Read the model definition and answer for the solid it produces. Units are mm, in the model's axes. Coordinates: 2 decimals unless noted, no trailing zeros. Order: outer loops, then holes, each group sorted by start corner. A loop starts at its lowest first (then second) coordinate and runs counter-clockwise, first axis right, second up. Notation, with made-up numbers: M 43,86 L 52,86 A28 cw 52,124 Z; hole C 40.25,3 d7. An arc over 180 degrees is marked long. One line per question, with ' | ' between items. Start each with the question number.
1) Find section D-D, the plane x = 5.75. Write down the section's boundary in (y, z).
2) Given P1, Ø4, axis at y = 4.5, z = -10, coming from the +X side; P2, Ø3, axis at x = -4.5, z = 9.5, coming from the -Y side; P3, Ø4, axis at y = 4, z = -4.5, coming from the -X side, each flat-ended and moving along its own axis, determine where each tip first touches the part or whether it passes through.
3) Find section B-B, the plane x = 0. Write down the section's boundary in (y, z), plus the area to 3 significant figures.
4) Find section C-C, the plane z = 10. Write down the section's boundary in (x, y), plus the area to 3 significant figures.
5) Consider probe 1 along Y at (x, z) = (0.9, -24); probe 2 along X at (y, z) = (1.5, 19); probe 3 along Z at (x, y) = (-0.25, 5.75). Determine where each line is inside the solid, lowest interval first.
6) Find section A-A, the plane z = -24. Write down the section's boundary in (x, y), plus the area to 3 significant figures.
from build123d import *

# Parameters (mm, degrees)
SKETCH1_W           = 4
SKETCH1_H           = 60
BOSS_EXTRUDE1_DEPTH = 8
SKETCH2_R           = 2.5
CUT_EXTRUDE1_DEPTH  = 8
FILLET1_R           = 3
SKETCH3_R           = 7.5
BOSS_EXTRUDE2_DEPTH = 4
BOSS_EXTRUDE3_DEPTH = 4


with BuildPart() as part:
    # Sketch1 → Boss-Extrude1 (new body)
    with BuildSketch(Plane(origin=(0, 0, 0), x_dir=(1, 0, 0), z_dir=(0, 1, 0))):
        Rectangle(SKETCH1_W, SKETCH1_H)
    extrude(amount=BOSS_EXTRUDE1_DEPTH)

    # Sketch2 → Cut-Extrude1 (cut)
    with BuildSketch(Plane.ZY.offset(2)):
        with Locations((-24, 4)):
            Circle(SKETCH2_R)
    extrude(amount=-CUT_EXTRUDE1_DEPTH, mode=Mode.SUBTRACT)

    # Fillet1
    fillet1_edges = [part.edges().sort_by_distance(p)[0] for p in [
        (0, 0, -30),
        (0, 8, -30),
    ]]
    fillet(fillet1_edges, radius=FILLET1_R)

    # Sketch3 → Boss-Extrude2 (add)
    with BuildSketch(Plane.XZ):
        with Locations((0, 30)):
            Circle(SKETCH3_R)
    extrude(amount=-BOSS_EXTRUDE2_DEPTH)

    # Sketch4 → Boss-Extrude3 (add)
    with BuildSketch(Plane(origin=(2, 0, 0), x_dir=(0, 0, -1), z_dir=(1, 0, 0))):
        Polygon((-30, 4), (-36.351721889, 4), (-30, 8), align=None)
    extrude(amount=-BOSS_EXTRUDE3_DEPTH)


solid = part.part
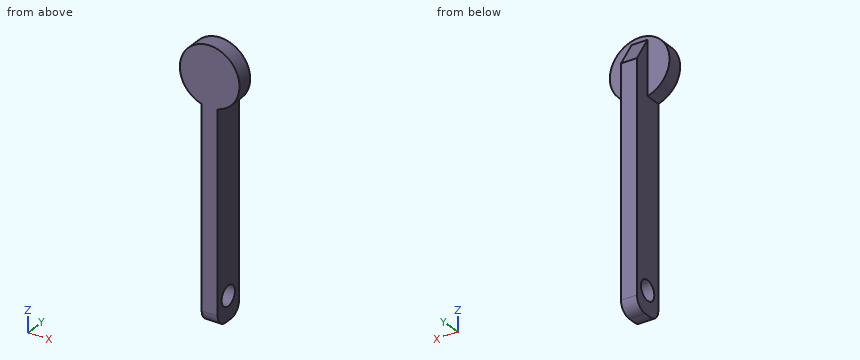
Report:
1) outline: M 0,25.18 L 4,25.18 L 4,34.82 L 0,34.82 Z
2) P1: stops at x = 2 | P2: passes through | P3: stops at x = -2
3) outline: M 0,-27 A3 ccw 3,-30 L 5,-30 A3 ccw 8,-27 L 8,30 L 4,36.35 L 4,37.5 L 0,37.5 Z; hole C 4,-24 d5 | area: 499 mm^2
4) outline: M -2,0 L 2,0 L 2,8 L -2,8 Z | area: 32.0 mm^2
5) probe 1: y = 0 to 1.5, 6.5 to 8 | probe 2: x = -2 to 2 | probe 3: z = -29.9 to -25.79, -22.21 to 33.57
6) outline: M -2,0 L 2,0 L 2,1.5 L -2,1.5 Z; M -2,6.5 L 2,6.5 L 2,8 L -2,8 Z | area: 12.0 mm^2
